Source: CAD feature listing. Evaluate the final solid. Frame: model axes, mm. A direction names the side the tool comes from. Round coordinates to 2 decimals unless told otherwise and drop trailing zeros. Order: outer loops, then holes, each group sorted by start corner. A loop starts at its lowest first (then second) coordinate and runs counter-clockwise, first axis right, second up. Notation, with made-up numbers: (37, 23) - (88, 23) arc R29 cw to (88, 61) - close; hole circle Ø2 at (3, 56). An arc over 180 degrees is marked (long way). Put each result on its own line as item: value. Start each with the question number.
1) Contact query for flat-ended pins moving along their axis: P1, Ø1.1, axis at x = -1.5, y = 0, coming from the -Z side; P2, Ø1.6, axis at x = -2.5, z = -6, coming from the +Y side; P3, Ø2, axis at y = -3, z = 7.5, coming from the -X side. Output: stop coordinate, or through.
2) Section A-A on z = 0. Output: boundary loops of the cut face in (x, y).
3) Mould query, pull axis Z, two halves, no side actions, for faces 4 (the face through (45.1, -2, -2)), 5 (the face through (33.61, -9.76, 2.17)), 6 (the face through (-4.099, 0.007, 6.865)), 7 (the face through (-4.099, 0.007, 5.435)). Classes: +Z half, -Z half, draft (parallel to the pull), parting line (faces both ways), or undercut.
4) Access query for faces 1 (the face through (39.442, 0.045, 6.476)), 2 (the face through (-4.099, 0.007, -5.435)), 3 (the face through (-2, 0.5, -6)). Directions: +Z, -Z, +X, -X, +Y, -Y. A direction counts if a zero-diameter tool reaches every point of the face in a straight line with its end or side. Return the directions, or none.
5) Section B-B on x = 43. Output: boundary loops of the cut face in (y, z).
6) Line query: probe 1 along Z at (x, y) = (1.5, 2); probe 2 along X at (y, z) = (-2.5, 4.25); probe 3 along Y at (x, z) = (38.4, 7.5) (3 decimals). Output: solid intervals per line, ascending. Write a range as [from, to].
7) Section C-C on x = 13. Output: boundary loops of the cut face in (y, z).
```python
from build123d import *

# Parameters (mm, degrees)
SKETCH1_R                          = 10.2
BOSS_EXTRUDE1_DEPTH                = 25.1
FILLET1_R                          = 1
SKETCH2_R                          = 10
BOSS_EXTRUDE2_DEPTH                = 17
FILLET2_R                          = 0.5
CHAMFER1_SIZE                      = 0.25
SKETCH3_R                          = 3.5
BOSS_EXTRUDE3_DEPTH                = 3
SKETCH4_R                          = 2
BOSS_EXTRUDE4_DEPTH                = 11
CUT_EXTRUDE1_DEPTH                 = 56.024449111
CUT_EXTRUDE1_DEPTH_BACK            = 56.024449111
M2_5X0_45_TAPPED_HOLE1_D           = 2.05
M2_5X0_45_TAPPED_HOLE1_DEPTH       = 5
M2_5X0_45_TAPPED_HOLE1_CSINK_D     = 2.55
M2_5X0_45_TAPPED_HOLE1_CSINK_ANGLE = 90
M2_5X0_45_TAPPED_HOLE1_TIP         = 0.615882135
SKETCH9_W                          = 2
SKETCH9_H                          = 1
BOSS_EXTRUDE5_DEPTH                = 4.4
FILLET3_R                          = 1


with BuildPart() as part:
    # Sketch1 → Boss-Extrude1 (new body)
    with BuildSketch(Plane(origin=(0, 0, 0), x_dir=(0, 0, -1), z_dir=(1, 0, 0))):
        Circle(SKETCH1_R)
    extrude(amount=BOSS_EXTRUDE1_DEPTH)

    # Fillet1
    fillet1_edges = [part.edges().sort_by_distance(p)[0] for p in [
        (25.1, 0, 10.2),
    ]]
    fillet(fillet1_edges, radius=FILLET1_R)

    # Sketch2 → Boss-Extrude2 (add)
    with BuildSketch(Plane(origin=(25.1, 0, 0), x_dir=(0, 0, -1), z_dir=(1, 0, 0))):
        Circle(SKETCH2_R)
    extrude(amount=BOSS_EXTRUDE2_DEPTH)

    # Fillet2
    fillet2_edges = [part.edges().sort_by_distance(p)[0] for p in [
        (25.1, 0, 10),
    ]]
    fillet(fillet2_edges, radius=FILLET2_R)

    # Chamfer1
    chamfer1_edges = [part.edges().sort_by_distance(p)[0] for p in [
        (0, 0, 10.2),
        (42.1, 0, 10),
    ]]
    chamfer(chamfer1_edges, length=CHAMFER1_SIZE)

    # Sketch3 → Boss-Extrude3 (add)
    with BuildSketch(Plane(origin=(42.1, 0, 0), x_dir=(0, 0, -1), z_dir=(1, 0, 0))):
        Circle(SKETCH3_R)
    extrude(amount=BOSS_EXTRUDE3_DEPTH)

    # Sketch4 → Boss-Extrude4 (add)
    with BuildSketch(Plane(origin=(42.1, 0, 0), x_dir=(0, 0, -1), z_dir=(1, 0, 0))):
        Circle(SKETCH4_R)
    extrude(amount=BOSS_EXTRUDE4_DEPTH)

    # Sketch6 → Cut-Extrude1 (cut, two sides: drawn at the far end of the back side and taken through both)
    with BuildSketch(Plane.XY.offset(-CUT_EXTRUDE1_DEPTH_BACK)):
        with BuildLine():
            Line((53.1, 2), (45.6, 2))
            ThreePointArc((45.6, 2), (45.746446609, 1.646446609), (46.1, 1.5))
            Line((46.1, 1.5), (53.1, 1.5))
            Line((53.1, 1.5), (53.1, 2))
        make_face()
    extrude(amount=CUT_EXTRUDE1_DEPTH + CUT_EXTRUDE1_DEPTH_BACK, mode=Mode.SUBTRACT)

    # M2.5x0.45 Tapped Hole1
    with Locations(Plane(origin=(42.1, 0, 0), x_dir=(0, 0, -1), z_dir=(1, 0, 0))):
        with Locations((-7.5, 0), (7.5, 0)):
            CounterSinkHole(M2_5X0_45_TAPPED_HOLE1_D / 2, M2_5X0_45_TAPPED_HOLE1_CSINK_D / 2, depth=M2_5X0_45_TAPPED_HOLE1_DEPTH, counter_sink_angle=M2_5X0_45_TAPPED_HOLE1_CSINK_ANGLE)
            with Locations((0, 0, -(M2_5X0_45_TAPPED_HOLE1_DEPTH + M2_5X0_45_TAPPED_HOLE1_TIP / 2))):  # 118° drill point
                Cone(0, M2_5X0_45_TAPPED_HOLE1_D / 2, M2_5X0_45_TAPPED_HOLE1_TIP, mode=Mode.SUBTRACT)

    # Sketch9 → Boss-Extrude5 (add)
    with BuildSketch(Plane.ZY):
        with Locations((-6.15, 0)):
            Rectangle(SKETCH9_W, SKETCH9_H)
        with Locations((6.15, 0)):
            Rectangle(SKETCH9_W, SKETCH9_H)
    extrude(amount=BOSS_EXTRUDE5_DEPTH)

    # Fillet3
    fillet3_edges = [part.edges().sort_by_distance(p)[0] for p in [
        (-4.4, 0, 7.15),
        (-4.4, 0, 5.15),
        (-4.4, 0, -5.15),
        (-4.4, 0, -7.15),
    ]]
    fillet(fillet3_edges, radius=FILLET3_R - 0.0001)  # a hair under: the kernel refuses the full size


solid = part.part
```
Answer sheet:
1. P1: z = -7.15
1. P2: y = 0.5
1. P3: x = 0
2. outline: (0, -9.95) - (0.25, -10.2) - (24.1, -10.2) arc R1 ccw to (25.1, -9.2) - (25.1, -9.5) arc R0.5 ccw to (25.6, -10) - (41.85, -10) - (42.1, -9.75) - (42.1, -3.5) - (45.1, -3.5) - (45.1, -2) - (53.1, -2) - (53.1, 1.5) - (46.1, 1.5) arc R0.5 cw to (45.6, 2) - (45.1, 2) - (45.1, 3.5) - (42.1, 3.5) - (42.1, 9.75) - (41.85, 10) - (25.6, 10) arc R0.5 ccw to (25.1, 9.5) - (25.1, 9.2) arc R1 ccw to (24.1, 10.2) - (0.25, 10.2) - (0, 9.95) - close
3. face 4: draft
3. face 5: parting line
3. face 6: +Z half
3. face 7: undercut
4. face 1: +X
4. face 2: -X, +Y, -Y
4. face 3: +Z, -Z, -X, +Y
5. outline: circle Ø7 at (0, 0)
6. probe 1: [-10, 10]
6. probe 2: [0, 42.1]
6. probe 3: [-6.614, -1.025], [1.025, 6.614]
7. outline: circle Ø20.4 at (0, 0)
